The model under review builds one solid part; all positions refer to its coordinate system, in mm. A direction names the side the tool comes from. Round coordinates to 2 decimals unless told otherwise and drop trailing zeros. Order: outer loops, then holes, each group sorted by start corner. A loop starts at its lowest first (then second) coordinate and runs counter-clockwise, first axis right, second up.
1) To check wall thickness, follow L1, parallel to Z at x = 2.25, y = 4.75; L2, parallel to Y at x = 3.25, z = -2; L3, parallel to Y at x = 2.8, z = -3.81. State the ranges of each line that lie inside material, in increasing order.
2) Mouldability with a two-part tool opening along Y and no side actions: class faces 1 (the face through (1.61, 4.94, -0.01)), 2 (the face through (2, -8.85, 0)), 3 (the face through (1.878, 4.424, 2.034)) as pulls with the +Y half, pulls with the -Y half, needs draft (parallel to the pull), parting line crosses it, or undercut.
3) Consider section D-D (z = 5). Give the boundary of the cut face in (x, y).
4) Clearance check with a flat-ended pin moving along its axis: P1, Ø4, axis at y = -6.31, z = -3.81, coming from the -X side. State where the tip first meets the part, or that it passes through.
5) Consider section B-B (z = 3). Give the boundary of the cut face in (x, y).
6) Consider section A-A (y = 5.5). Give the boundary of the cut face in (x, z) (3 decimals), then the cut area to 3 significant figures.
7) Consider section C-C (y = 0). Give the boundary of the cut face in (x, z).
8) Machinability: for faces 4 (the face through (3.63, 7.64, -0.08)), 5 (the face through (3.13, 0.06, -1.35)), which of the approach directions +Z, -Z, +X, -X, +Y, -Y give a long, thin tool a straight path to every point of the face, cutting with its end or side? Answer none if there is none.
from build123d import *

# Parameters (mm, degrees)
BOSS_EXTRUDE1_DEPTH            = 6.35
F_8_32_TAPPED_HOLE1_D          = 3.4544
F_8_32_TAPPED_HOLE1_DEPTH      = 3.048
F_8_32_TAPPED_HOLE1_TIP        = 1.037806461
F_6_32_TAPPED_HOLE1_D          = 2.7051
F_6_32_TAPPED_HOLE1_DEPTH      = 9.398
F_6_32_TAPPED_HOLE1_TIP        = 0.81269403
F_6_0_204_DIAMETER_HOLE1_DEPTH = 3.81


# Read off the part's stored shape, not the designer's step: #6 (0.204) Diameter Hole1
with BuildPart() as part:
    # Sketch1 → Boss-Extrude1 (new, symmetric)
    with BuildSketch(Plane.XY):
        with BuildLine():
            ThreePointArc((0, -2.499995), (2.499995, 0), (0, 2.499995))
            Line((0, 2.499995), (0, 8.849995))
            Line((0, 8.849995), (3.81, 8.849995))
            Line((3.81, 8.849995), (3.81, -8.849995))
            Line((3.81, -8.849995), (0, -8.849995))
            Line((0, -8.849995), (0, -2.499995))
        make_face()
    extrude(amount=BOSS_EXTRUDE1_DEPTH, both=True)

    # #8-32 Tapped Hole1
    with Locations(Plane(origin=(0, 8.849995, 0), x_dir=(1, 0, 0), z_dir=(0, 1, 0))):
        with Locations((1.905, 0)):
            Hole(F_8_32_TAPPED_HOLE1_D / 2, depth=F_8_32_TAPPED_HOLE1_DEPTH)
            with Locations((0, 0, -(F_8_32_TAPPED_HOLE1_DEPTH + F_8_32_TAPPED_HOLE1_TIP / 2))):  # 118° drill point
                Cone(0, F_8_32_TAPPED_HOLE1_D / 2, F_8_32_TAPPED_HOLE1_TIP, mode=Mode.SUBTRACT)

    # #6-32 Tapped Hole1
    with Locations(Plane(origin=(3.81, 0, 0), x_dir=(0, 0, -1), z_dir=(1, 0, 0))):
        with Locations((0, 0)):
            Hole(F_6_32_TAPPED_HOLE1_D / 2, depth=F_6_32_TAPPED_HOLE1_DEPTH)
            with Locations((0, 0, -(F_6_32_TAPPED_HOLE1_DEPTH + F_6_32_TAPPED_HOLE1_TIP / 2))):  # 118° drill point
                Cone(0, F_6_32_TAPPED_HOLE1_D / 2, F_6_32_TAPPED_HOLE1_TIP, mode=Mode.SUBTRACT)

    # #6 (0.204) Diameter Hole1 outline → #6 (0.204) Diameter Hole1 (cut)
    with BuildSketch(Plane.YZ):
        with BuildLine():
            Line((-8.849995, 6.35), (-8.849995, 3.299466318))
            ThreePointArc((-8.849995, 3.299466318), (-4.478022751, 1.978027751), (-5.799461318, 6.35))
            Line((-5.799461318, 6.35), (-8.849995, 6.35))
        make_face()
        with BuildLine():
            ThreePointArc((-5.799461318, -6.35), (-4.478022751, -1.978027751), (-8.849995, -3.299466318))
            Line((-8.849995, -3.299466318), (-8.849995, -6.35))
            Line((-8.849995, -6.35), (-5.799461318, -6.35))
        make_face()
        with BuildLine():
            Line((8.849995, 6.35), (5.799461318, 6.35))
            ThreePointArc((5.799461318, 6.35), (4.478022751, 1.978027751), (8.849995, 3.299466318))
            Line((8.849995, 3.299466318), (8.849995, 6.35))
        make_face()
        with BuildLine():
            ThreePointArc((8.849995, -3.299466318), (4.478022751, -1.978027751), (5.799461318, -6.35))
            Line((5.799461318, -6.35), (8.849995, -6.35))
            Line((8.849995, -6.35), (8.849995, -3.299466318))
        make_face()
    extrude(amount=F_6_0_204_DIAMETER_HOLE1_DEPTH, mode=Mode.SUBTRACT)


solid = part.part
Answer below:
1. L1: z = -6.35 to -5.88, -1.74 to 1.74, 5.88 to 6.35
1. L2: y = -8.85 to -8.16, -4.46 to 4.46, 8.16 to 8.85
1. L3: y = -3.72 to 3.72
2. face 1: pulls with the +Y half
2. face 2: pulls with the -Y half
2. face 3: undercut
3. outline: (0, -4.01) - (3.81, -4.01) - (3.81, 4.01) - (0, 4.01) - (0, 2.5) arc R2.5 cw to (0, -2.5) - close
4. P1: passes through
5. outline: (0, -8.85) - (3.81, -8.85) - (3.81, -8.77) - (0, -8.77) - close; (0, -3.85) - (3.81, -3.85) - (3.81, 3.85) - (0, 3.85) - (0, 2.5) arc R2.5 cw to (0, -2.5) - close; (0, 8.77) - (3.81, 8.77) - (3.81, 8.85) - (0, 8.85) - close
6. outline: (0, -6.35) - (3.81, -6.35) - (3.81, -6.271) - (0, -6.271) - close; (0, -1.349) - (3.81, -1.349) - (3.81, 1.349) - (0, 1.349) - close; (0, 6.271) - (3.81, 6.271) - (3.81, 6.35) - (0, 6.35) - close; hole circle Ø2.449 at (1.905, 0)
6. area: 6.17 mm2
7. outline: (2.5, -6.35) - (3.81, -6.35) - (3.81, -1.35) - (2.5, -1.35) - close; (2.5, 1.35) - (3.81, 1.35) - (3.81, 6.35) - (2.5, 6.35) - close
8. face 4: +Y
8. face 5: +X, -X
